The drawing under review shows one solid part. Ordinate dimensions are in mm from its lowest x, y, z. A direction names the side the tool comes from. Coordinates: 2 decimals unless noted, no trailing zeros. Order: outer loops, then holes, each group sorted by start corner. A loop starts at its lowest first (then second) coordinate and runs counter-clockwise, first axis right, second up.
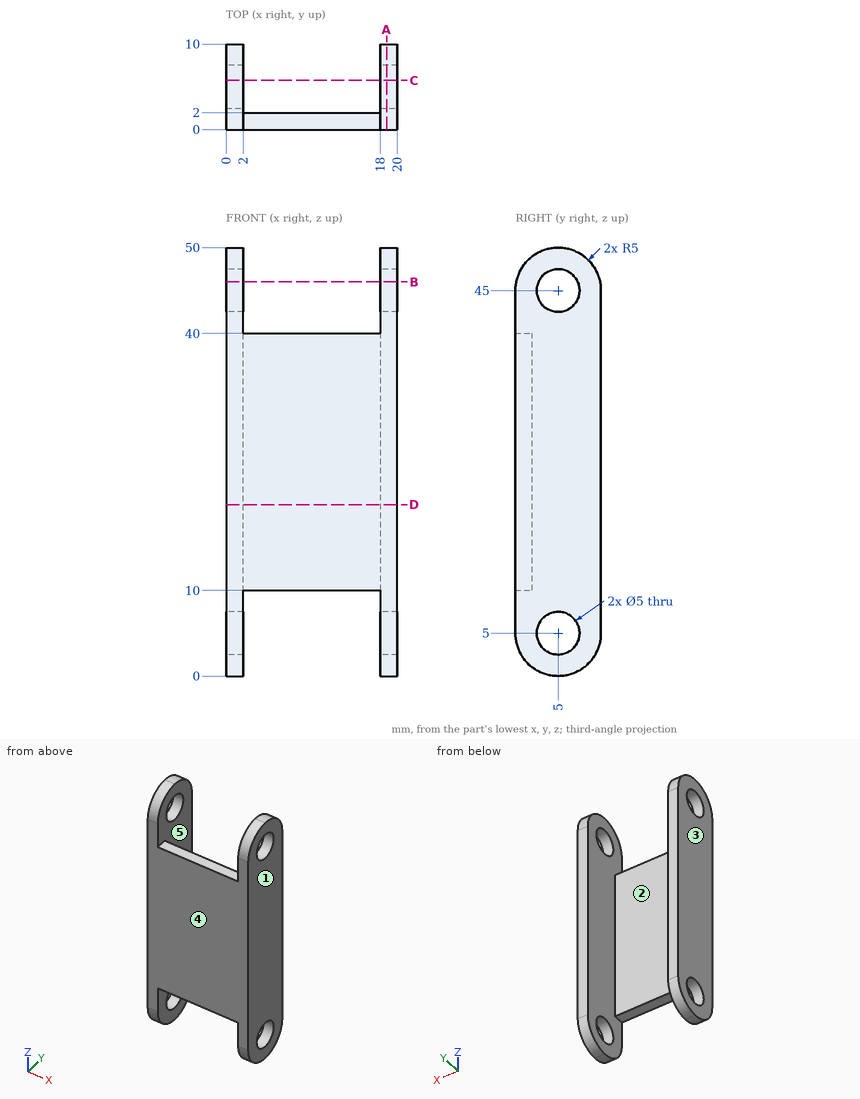
(1) Wall thickness on probe 1 along Z at (x, y) = (18.7, 5); probe 2 along X at (y, z) = (4.75, 20.5); probe 3 along Y at (x, z) = (18.4, 5): over which ranges is each line inside the solid? List them lowest first.
A:
probe 1: z = 0 to 2.5, 7.5 to 42.5, 47.5 to 50
probe 2: x = 0 to 2, 18 to 20
probe 3: y = 0 to 2.5, 7.5 to 10
(2) We need section B-B, the plane z = 46. Write out the cut boundary in (x, y), and give its area (3 significant figures).
A:
outline: (0, 0.1) - (2, 0.1) - (2, 2.71) - (0, 2.71) - close; (0, 7.29) - (2, 7.29) - (2, 9.9) - (0, 9.9) - close; (18, 0.1) - (20, 0.1) - (20, 2.71) - (18, 2.71) - close; (18, 7.29) - (20, 7.29) - (20, 9.9) - (18, 9.9) - close
area: 20.9 mm2
(3) For pin 1 Ø1 at (x, y) = (6, 1) entering from -Z; pin 2 Ø0.6 at (x, y) = (11, 1) entering from +Z, all flat-tipped, find the tip position at first contact; note any pin that passes through.
A:
pin 1: stops at z = 10
pin 2: stops at z = 40
(4) We need section D-D, the plane z = 20. Write out the cut boundary in (x, y).
A:
outline: (0, 0) - (20, 0) - (20, 10) - (18, 10) - (18, 2) - (2, 2) - (2, 10) - (0, 10) - close
(5) Machinability: for the marked faces 1 and 2, which of the approach directions +Z, -Z, +X, -X, +Y, -Y give a long, thin tool a straight path to every point of the face, cutting with its end or side? Answer none if there is none.
A:
face 1: +Z, -Z, +X, +Y, -Y
face 2: +Z, -Z, +Y
(6) Draft analysis for pull direction X (two halves, no side actions). For the marked faces 3, 4 and 5, state which applies: released by +X, released by -X, zero draft, split by the parting line, or undercut.
A:
face 3: released by -X
face 4: zero draft
face 5: undercut
(7) We need section A-A, the plane x = 18.75. Write out the cut boundary in (y, z).
A:
outline: (0, 5) arc R5 ccw to (10, 5) - (10, 45) arc R5 ccw to (0, 45) - close; hole circle Ø5 at (5, 5); hole circle Ø5 at (5, 45)
(8) We need section C-C, the plane y = 5.75. Write out the cut boundary in (x, z), and give its area (3 significant figures).
A:
outline: (0, 0.06) - (2, 0.06) - (2, 2.62) - (0, 2.62) - close; (0, 7.38) - (2, 7.38) - (2, 42.62) - (0, 42.62) - close; (0, 47.38) - (2, 47.38) - (2, 49.94) - (0, 49.94) - close; (18, 0.06) - (20, 0.06) - (20, 2.62) - (18, 2.62) - close; (18, 7.38) - (20, 7.38) - (20, 42.62) - (18, 42.62) - close; (18, 47.38) - (20, 47.38) - (20, 49.94) - (18, 49.94) - close
area: 161 mm2
